from build123d import *

# Parameters (mm, degrees)
SKETCH_1_W               = 34
SKETCH_1_H               = 34
SKETCH_1_R               = 16.25
SKETCH_1_R_2             = 1.75
SKETCH_1_R_3             = 1.5
EXTRUDE_1_DEPTH          = 5
SKETCH_2_W               = 34
SKETCH_2_H               = 3
EXTRUDE_2_DEPTH          = 12
SKETCH_5_R               = 1.5
CUT_EXTRUDE_4_DEPTH      = 29.861739379
SKETCH_16_W              = 34
SKETCH_16_H              = 10
EXTRUDE_4_DEPTH          = 5
SKETCH_17_W              = 39
SKETCH_17_H              = 5
EXTRUDE_5_DEPTH          = 5
SKETCH_20_W              = 5
SKETCH_20_H              = 39
EXTRUDE_6_DEPTH          = 5
SKETCH_22_W              = 5
SKETCH_22_H              = 39
EXTRUDE_7_DEPTH          = 5
SKETCH_25_W              = 34
SKETCH_25_H              = 3
EXTRUDE_8_DEPTH          = 12
SKETCH_26_W              = 3
SKETCH_26_H              = 24
EXTRUDE_9_DEPTH          = 10
FILLET_1_R               = 5
FILLET_2_R               = 5
SKETCH_27_R              = 1.5
CUT_EXTRUDE_10_DEPTH     = 49.928519291
SKETCH_29_R              = 2
CUT_EXTRUDE_11_DEPTH     = 1
MIRROR_4_COPY_1_SKETCH_R = 1.5
MIRROR_4_COPY_1_DEPTH    = 49.928519291
MIRROR_4_COPY_2_SKETCH_R = 2
MIRROR_4_COPY_2_DEPTH    = 1


with BuildPart() as part:
    # 草图1 → 凸台-拉伸1 (new, symmetric)
    with BuildSketch(Plane(origin=(0, 0, 0), x_dir=(1, 0, 0), z_dir=(0, 1, 0))):
        Rectangle(SKETCH_1_W, SKETCH_1_H)
        with Locations(Location((0, 0, 0), (0, 0, 270))):
            Circle(SKETCH_1_R, mode=Mode.SUBTRACT)
        with Locations(Location((13.258252147, 13.258252147, 0), (0, 0, 270))):
            Circle(SKETCH_1_R_2, mode=Mode.SUBTRACT)
        with Locations(Location((13.258252147, -13.258252147, 0), (0, 0, 270))):
            Circle(SKETCH_1_R_3, mode=Mode.SUBTRACT)
        with Locations(Location((-13.258252147, 13.258252147, 0), (0, 0, 270))):
            Circle(SKETCH_1_R_3, mode=Mode.SUBTRACT)
        with Locations(Location((-13.258252147, -13.258252147, 0), (0, 0, 270))):
            Circle(SKETCH_1_R_2, mode=Mode.SUBTRACT)
    extrude(amount=EXTRUDE_1_DEPTH, both=True)

    # 草图2 → 凸台-拉伸2 (add)
    with BuildSketch(Plane(origin=(0, 0, 0), x_dir=(1, 0, 0), z_dir=(0, 1, 0))):
        with Locations((0, -18.5)):
            Rectangle(SKETCH_2_W, SKETCH_2_H)
    extrude(amount=EXTRUDE_2_DEPTH)

    # 草图5 → 切除-拉伸4 (cut, through all)
    with BuildSketch(Plane.XY):
        with Locations((-8.5, 9)):
            Circle(SKETCH_5_R)
        with Locations(Location((8.5, 9, 0), (0, 0, 180))):
            Circle(SKETCH_5_R)
    extrude(amount=CUT_EXTRUDE_4_DEPTH, mode=Mode.SUBTRACT)

    # 草图16 → 凸台-拉伸4 (add)
    with BuildSketch(Plane(origin=(0, 0, -17), x_dir=(-1, 0, 0), z_dir=(0, 0, -1))):
        Rectangle(SKETCH_16_W, SKETCH_16_H)
    extrude(amount=EXTRUDE_4_DEPTH)

    # 草图17 → 凸台-拉伸5 (add)
    with BuildSketch(Plane.ZY.offset(17)):
        with Locations((-2.5, 2.5)):
            Rectangle(SKETCH_17_W, SKETCH_17_H)
    extrude_5 = extrude(amount=EXTRUDE_5_DEPTH)

    # 镜向1: 凸台-拉伸5 across plane
    add(extrude_5.mirror(Plane(origin=(0, 0, 0), x_dir=(0, 0, 1), z_dir=(1, 0, 0))))

    # 草图20 → 凸台-拉伸6 (add, symmetric)
    with BuildSketch(Plane.XZ):
        with Locations((-19.5, -2.5)):
            Rectangle(SKETCH_20_W, SKETCH_20_H)
    extrude(amount=EXTRUDE_6_DEPTH, both=True)

    # 草图22 → 凸台-拉伸7 (add, symmetric)
    with BuildSketch(Plane.XZ):
        with Locations((19.5, -2.5)):
            Rectangle(SKETCH_22_W, SKETCH_22_H)
    extrude(amount=EXTRUDE_7_DEPTH, both=True)

    # 草图25 → 凸台-拉伸8 (add, symmetric)
    with BuildSketch(Plane.XZ):
        with Locations((0, 18.5)):
            Rectangle(SKETCH_25_W, SKETCH_25_H)
    extrude(amount=EXTRUDE_8_DEPTH, both=True)

    # 草图26 → 凸台-拉伸9 (add)
    with BuildSketch(Plane.ZY.offset(17)):
        with Locations((18.5, 0)):
            Rectangle(SKETCH_26_W, SKETCH_26_H)
    extrude_9 = extrude(amount=EXTRUDE_9_DEPTH)

    # 镜向2: 凸台-拉伸9 across plane
    add(extrude_9.mirror(Plane(origin=(0, 0, 0), x_dir=(0, 0, 1), z_dir=(1, 0, 0))))

    # 圆角1
    fillet_1_edges = [part.edges().sort_by_distance(p)[0] for p in [
        (-22, 0, -22),
        (22, 0, -22),
    ]]
    fillet(fillet_1_edges, radius=FILLET_1_R)

    # 圆角2
    fillet_2_edges = [part.edges().sort_by_distance(p)[0] for p in [
        (-27, -12, 18.5),
        (-27, 12, 18.5),
        (27, 12, 18.5),
        (27, -12, 18.5),
    ]]
    fillet(fillet_2_edges, radius=FILLET_2_R)

    # 草图27 → 切除-拉伸10 (cut, through all)
    with BuildSketch(Plane(origin=(0, 0, 17), x_dir=(-1, 0, 0), z_dir=(0, 0, -1))):
        with Locations((8.5, -9)):
            Circle(SKETCH_27_R)
    cut_extrude_10 = extrude(amount=-CUT_EXTRUDE_10_DEPTH, mode=Mode.SUBTRACT)

    # 草图29 → 切除-拉伸11 (cut)
    with BuildSketch(Plane(origin=(0, 0, 17), x_dir=(-1, 0, 0), z_dir=(0, 0, -1))):
        with Locations((8.5, -9)):
            Circle(SKETCH_29_R)
    cut_extrude_11 = extrude(amount=-CUT_EXTRUDE_11_DEPTH, mode=Mode.SUBTRACT)

    # 镜向3: 切除-拉伸10, 切除-拉伸11 across plane
    add(cut_extrude_10.mirror(Plane(origin=(0, 0, 0), x_dir=(0, 0, 1), z_dir=(1, 0, 0))), mode=Mode.SUBTRACT)
    add(cut_extrude_11.mirror(Plane(origin=(0, 0, 0), x_dir=(0, 0, 1), z_dir=(1, 0, 0))), mode=Mode.SUBTRACT)

    # 镜向4: 切除-拉伸10, 切除-拉伸11 across plane
    add(cut_extrude_10.mirror(Plane.ZX), mode=Mode.SUBTRACT)
    add(cut_extrude_11.mirror(Plane.ZX), mode=Mode.SUBTRACT)

    # 镜向4 copy 1 sketch → 镜向4 copy 1 (cut, through all)
    with BuildSketch(Plane(origin=(0, 0, 17), x_dir=(1, 0, 0), z_dir=(0, 0, -1))):
        with Locations((8.5, -9)):
            Circle(MIRROR_4_COPY_1_SKETCH_R)
    extrude(amount=-MIRROR_4_COPY_1_DEPTH, mode=Mode.SUBTRACT)

    # 镜向4 copy 2 sketch → 镜向4 copy 2 (cut)
    with BuildSketch(Plane(origin=(0, 0, 17), x_dir=(1, 0, 0), z_dir=(0, 0, -1))):
        with Locations((8.5, -9)):
            Circle(MIRROR_4_COPY_2_SKETCH_R)
    extrude(amount=-MIRROR_4_COPY_2_DEPTH, mode=Mode.SUBTRACT)


solid = part.part
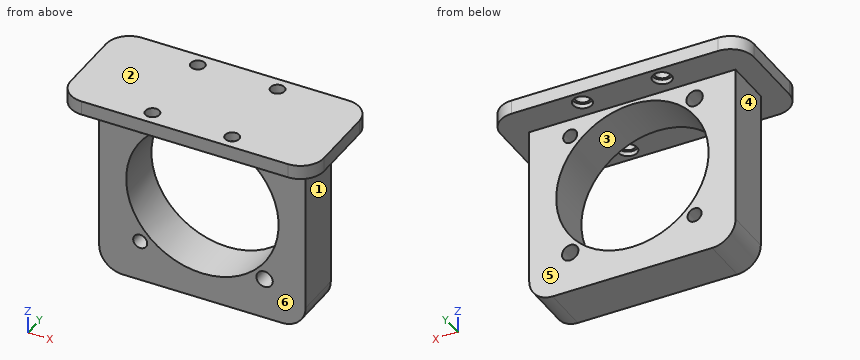
Work out the finished part from the listing and answer in its coordinate system (mm). Face numbers are marked on the shaded views. A direction names the side the tool comes from. Give positions to 0.01 mm unless a question says otherwise; leave off trailing zeros. Loops run counter-clockwise (first coordinate to the right, second up) from the corner with the lowest first, then second, coordinate; pieces in that order, holes last. Notation, with made-up numbers: M 49,47.25 L 100,47.25 A23 ccw 100,86.25 Z; hole C 54,-18 d6. An arc over 180 degrees is marked long. Use CSV: the item, a comma, the result in double quotes.
1) Determine the mould class of the marked faces 1, 2 and 3 for opening direction X: released by +X, released by -X, zero draft, split by the parting line, or undercut.
Answer:
face 1,"released by +X"
face 2,"zero draft"
face 3,"undercut"
2) Find section B-B on z = 7. Write down the section's boundary in (x, y) (3 decimals), plus the area to 3 significant figures.
Answer:
outline,"M -22,-5 L -14.665,-5 L -14.665,5 L -22,5 Z; M 14.665,-5 L 22,-5 L 22,5 L 14.665,5 Z"
area,"147 mm^2"
3) Given P1, Ø5, axis at x = -8.5, y = 9, coming from the -Z side; P2, Ø8, axis at y = 1.5, z = -5.5, coming from the -X side; P3, Ø12, axis at x = -19, z = 6.5, coming from the -Y side, each flat-ended and moving along its own axis, determine where each tip first touches the part or whether it passes through.
Answer:
P1,"z = 17"
P2,"x = -22"
P3,"y = -5"
4) Which of the six approach directions +Z, -Z, +X, -X, +Y, -Y give full straight-line access (tool end or side, diameter ignored) to the marked faces 4, 5 and 6?
Answer:
face 4,"-Z, -X, +Y, -Y"
face 5,"-Z, +X, -X, +Y"
face 6,"-Z, +X, -X, -Y"
5) Consider L1, parallel to Y at x = 8.5, z = 17.25; L2, parallel to Y at x = 8.5, z = 18.6; L3, parallel to Y at x = -18, z = 14. Determine where each line is inside the solid, lowest interval first.
Answer:
L1,"-12 to -11, -7 to 7, 11 to 12"
L2,"-12 to -10.5, -7.5 to 7.5, 10.5 to 12"
L3,"-5 to 5"
6) Find section C-C on x = 21. Write down the section's boundary in (y, z), plus the area to 3 significant figures.
Answer:
outline,"M -12,17 L -5,17 L -5,-20 L 5,-20 L 5,17 L 12,17 L 12,20 L -12,20 Z"
area,"442 mm^2"
7) Find section A-A on x = 0. Write down the section's boundary in (y, z).
Answer:
outline,"M -12,17 L -5,17 L -5,16.25 L 5,16.25 L 5,17 L 12,17 L 12,20 L -12,20 Z; M -5,-22 L 5,-22 L 5,-16.25 L -5,-16.25 Z"
8) Find section D-D on y = 3. Write down the section's boundary in (x, z), plus the area to 3 significant figures.
Answer:
outline,"M -27,17 L -22,17 L -22,-17 A5 ccw -17,-22 L 17,-22 A5 ccw 22,-17 L 22,17 L 27,17 L 27,20 L -27,20 Z; hole C 0,0 d32.5; hole C -13.26,13.26 d3.5; hole C -13.26,-13.26 d3; hole C 13.26,-13.26 d3.5; hole C 13.26,13.26 d3"
area,"1,000 mm^2"
